from build123d import *

# Parameters (mm, degrees)
EXTRUDE1_DEPTH  = 5
SKETCH3_W       = 42
SKETCH3_H       = 47
EXTRUDE2_DEPTH  = 5
SKETCH4_W       = 34
SKETCH4_H       = 40
EXTRUDE3_DEPTH  = 3.2
EXTRUDE4_DEPTH  = 3
SKETCH6_R       = 1.5
EXTRUDE5_DEPTH  = 5
SKETCH7_R       = 1.5
EXTRUDE6_DEPTH  = 5
SKETCH8_W       = 6.381599337
SKETCH8_H       = 7
EXTRUDE7_DEPTH  = 5
SKETCH9_R       = 1.5
EXTRUDE8_DEPTH  = 5
FILLET1_R       = 5
FILLET2_R       = 2
SKETCH11_R      = 2
EXTRUDE10_DEPTH = 5
SKETCH15_R      = 13
EXTRUDE13_DEPTH = 4
SKETCH16_W      = 45
SKETCH16_H      = 40
EXTRUDE14_DEPTH = 3.5
SKETCH17_R      = 1.5
EXTRUDE16_DEPTH = 5
SKETCH18_R      = 1.5
EXTRUDE17_DEPTH = 5
SKETCH20_R      = 2
EXTRUDE19_DEPTH = 5
EXTRUDE24_START = -1.5
EXTRUDE24_DEPTH = 1.5
EXTRUDE25_START = -1.5
EXTRUDE25_DEPTH = 1.5
SKETCH27_R      = 1.5
EXTRUDE26_DEPTH = 5
SKETCH28_R      = 1.5
EXTRUDE27_DEPTH = 5
SKETCH29_R      = 4
EXTRUDE28_DEPTH = 3
SKETCH30_R      = 2
EXTRUDE29_DEPTH = 2
SKETCH14_R      = 1.25
EXTRUDE30_DEPTH = 5


with BuildPart() as part:
    # Sketch2 → Extrude1 (new body)
    with BuildSketch(Plane(origin=(0, 0, 0), x_dir=(1, 0, 0), z_dir=(0, 1, 0))):
        with BuildLine():
            Line((82.558104656, 20.227687844), (67.247468193, 10.284844268))
            Line((67.247468193, 10.284844268), (38.381599337, 54.73438437))
            Line((38.381599337, 54.73438437), (38.381599337, 66.73438437))
            Line((38.381599337, 66.73438437), (-38.381599337, 66.73438437))
            Line((-38.381599337, 66.73438437), (-38.381599337, 54.73438437))
            Line((-38.381599337, 54.73438437), (-67.247468193, 10.284844268))
            Line((-67.247468193, 10.284844268), (-82.558104656, 20.227687844))
            ThreePointArc((-82.558104656, 20.227687844), (-84.534361106, -8.884919378), (-76.54843921, -36.950459463))
            Line((-76.54843921, -36.950459463), (-63.639610307, -24.04163056))
            Line((-63.639610307, -24.04163056), (-24.04163056, -63.639610307))
            Line((-24.04163056, -63.639610307), (-36.950459463, -76.54843921))
            ThreePointArc((-36.950459463, -76.54843921), (0, -85), (36.950459463, -76.54843921))
            Line((36.950459463, -76.54843921), (24.04163056, -63.639610307))
            Line((24.04163056, -63.639610307), (63.639610307, -24.04163056))
            Line((63.639610307, -24.04163056), (76.54843921, -36.950459463))
            ThreePointArc((76.54843921, -36.950459463), (84.534361106, -8.884919378), (82.558104656, 20.227687844))
        make_face()
    extrude(amount=-EXTRUDE1_DEPTH)

    # Sketch3 → Extrude2 (cut)
    with BuildSketch(Plane(origin=(0, 0, 0), x_dir=(1, 0, 0), z_dir=(0, 1, 0))):
        with Locations((0, 48.23438437)):
            Rectangle(SKETCH3_W, SKETCH3_H)
    extrude(amount=-EXTRUDE2_DEPTH, mode=Mode.SUBTRACT)

    # Sketch4 → Extrude3 (cut)
    with BuildSketch(Plane(origin=(0, 0, 0), x_dir=(-1, 0, 0), z_dir=(0, 1, 0))):
        with Locations((0, -10.73438437)):
            Rectangle(SKETCH4_W, SKETCH4_H)
    extrude(amount=-EXTRUDE3_DEPTH, mode=Mode.SUBTRACT)

    # Sketch5 → Extrude4 (cut)
    with BuildSketch(Plane(origin=(0, 0, 0), x_dir=(1, 0, 0), z_dir=(0, 1, 0))):
        Polygon((43.470660758, -6.348358315), (62.76008382, 6.17833949), (43.697717595, 35.531809369), (24.408294532, 23.005111563), align=None)
    extrude4 = extrude(amount=-EXTRUDE4_DEPTH, mode=Mode.SUBTRACT)

    # Mirror1: Extrude4 across plane
    add(extrude4.mirror(Plane(origin=(0, 0, 0), x_dir=(0, 0, 1), z_dir=(1, 0, 0))), mode=Mode.SUBTRACT)

    # Sketch6 → Extrude5 (cut)
    with BuildSketch(Plane(origin=(0, 0, 0), x_dir=(1, 0, 0), z_dir=(0, 1, 0))):
        with Locations(Location((42.401256054, 43.036420449, 0), (0, 0, 270))):
            Circle(SKETCH6_R)
        with Locations(Location((60.918983244, 14.521621139, 0), (0, 0, 270))):
            Circle(SKETCH6_R)
        with Locations(Location((50.911688245, -32.526911935, 0), (0, 0, 270))):
            Circle(SKETCH6_R)
        with Locations(Location((32.526911935, -50.911688245, 0), (0, 0, 270))):
            Circle(SKETCH6_R)
    extrude5 = extrude(amount=-EXTRUDE5_DEPTH, mode=Mode.SUBTRACT)

    # Mirror2: Extrude5 across plane
    add(extrude5.mirror(Plane(origin=(0, 0, 0), x_dir=(0, 0, 1), z_dir=(1, 0, 0))), mode=Mode.SUBTRACT)

    # Sketch7 → Extrude6 (cut)
    with BuildSketch(Plane(origin=(0, 0, 0), x_dir=(-1, 0, 0), z_dir=(0, 1, 0))):
        with Locations(Location((-24, -63.73438437, 0), (0, 0, 90))):
            Circle(SKETCH7_R)
        with Locations(Location((-24, -27.73438437, 0), (0, 0, 90))):
            Circle(SKETCH7_R)
    extrude6 = extrude(amount=-EXTRUDE6_DEPTH, mode=Mode.SUBTRACT)

    # Mirror3: Extrude6 across plane
    add(extrude6.mirror(Plane(origin=(0, 0, 0), x_dir=(0, 0, 1), z_dir=(1, 0, 0))), mode=Mode.SUBTRACT)

    # Sketch8 → Extrude7 (cut)
    with BuildSketch(Plane(origin=(0, 0, 0), x_dir=(1, 0, 0), z_dir=(0, 1, 0))):
        with Locations((30.190799669, 65.23438437)):
            Rectangle(SKETCH8_W, SKETCH8_H)
    extrude7 = extrude(amount=-EXTRUDE7_DEPTH, mode=Mode.SUBTRACT)

    # Mirror4: Extrude7 across plane
    add(extrude7.mirror(Plane(origin=(0, 0, 0), x_dir=(0, 0, 1), z_dir=(1, 0, 0))), mode=Mode.SUBTRACT)

    # Sketch9 → Extrude8 (cut)
    with BuildSketch(Plane(origin=(0, 0, 0), x_dir=(1, 0, 0), z_dir=(0, 1, 0))):
        with Locations(Location((35.881599337, 60.13438437, 0), (0, 0, 270))):
            Circle(SKETCH9_R)
        with Locations(Location((35.881599337, 46.73438437, 0), (0, 0, 270))):
            Circle(SKETCH9_R)
    extrude8 = extrude(amount=-EXTRUDE8_DEPTH, mode=Mode.SUBTRACT)

    # Mirror5: Extrude8 across plane
    add(extrude8.mirror(Plane(origin=(0, 0, 0), x_dir=(0, 0, 1), z_dir=(1, 0, 0))), mode=Mode.SUBTRACT)

    # Fillet1
    fillet1_edges = [part.edges().sort_by_distance(p)[0] for p in [
        (76.54843921, -2.5, 36.950459463),
        (63.639610307, -2.5, 24.04163056),
        (24.04163056, -2.5, 63.639610307),
        (36.950459463, -2.5, 76.54843921),
        (-36.950459463, -2.5, 76.54843921),
        (-24.04163056, -2.5, 63.639610307),
        (-63.639610307, -2.5, 24.04163056),
        (-76.54843921, -2.5, 36.950459463),
        (-82.558104656, -2.5, -20.227687844),
        (-67.247468193, -2.5, -10.284844268),
        (-38.381599337, -2.5, -54.73438437),
        (38.381599337, -2.5, -54.73438437),
        (67.247468193, -2.5, -10.284844268),
        (82.558104656, -2.5, -20.227687844),
    ]]
    fillet(fillet1_edges, radius=FILLET1_R)

    # Fillet2
    fillet2_edges = [part.edges().sort_by_distance(p)[0] for p in [
        (-43.470660758, -1.5, 6.348358315),
        (-62.76008382, -1.5, -6.17833949),
        (-43.697717595, -1.5, -35.531809369),
        (-17, -1.6, 9.26561563),
        (17, -1.6, 9.26561563),
        (43.470660758, -1.5, 6.348358315),
        (24.408294532, -1.5, -23.005111563),
        (43.697717595, -1.5, -35.531809369),
        (62.76008382, -1.5, -6.17833949),
        (-24.408294532, -1.5, -23.005111563),
    ]]
    fillet(fillet2_edges, radius=FILLET2_R)

    # Sketch11 → Extrude10 (cut)
    with BuildSketch(Plane(origin=(0, 0, 0), x_dir=(1, 0, 0), z_dir=(0, 1, 0))):
        with Locations(Location((24.5, 36, 0), (0, 0, 270))):
            Circle(SKETCH11_R)
        with Locations(Location((-24.5, 36, 0), (0, 0, 270))):
            Circle(SKETCH11_R)
    extrude(amount=-EXTRUDE10_DEPTH, mode=Mode.SUBTRACT)

    # Sketch15 → Extrude13 (cut)
    with BuildSketch(Plane(origin=(0, 0, 0), x_dir=(1, 0, 0), z_dir=(0, 1, 0))):
        with Locations(Location((69, -13, 0), (0, 0, 270))):
            Circle(SKETCH15_R)
    extrude13 = extrude(amount=-EXTRUDE13_DEPTH, mode=Mode.SUBTRACT)

    # Mirror7: Extrude13 across plane
    add(extrude13.mirror(Plane(origin=(0, 0, 0), x_dir=(0, 0, 1), z_dir=(1, 0, 0))), mode=Mode.SUBTRACT)

    # Sketch16 → Extrude14 (cut)
    with BuildSketch(Plane(origin=(0, 0, 0), x_dir=(1, 0, 0), z_dir=(0, 1, 0))):
        with Locations((0, -75)):
            Rectangle(SKETCH16_W, SKETCH16_H)
    extrude(amount=-EXTRUDE14_DEPTH, mode=Mode.SUBTRACT)

    # Sketch17 → Extrude16 (cut)
    with BuildSketch(Plane(origin=(0, 0, 0), x_dir=(1, 0, 0), z_dir=(0, 1, 0))):
        with Locations(Location((25.5, -70, 0), (0, 0, 270))):
            Circle(SKETCH17_R)
        with Locations(Location((-25.5, -70, 0), (0, 0, 270))):
            Circle(SKETCH17_R)
    extrude(amount=-EXTRUDE16_DEPTH, mode=Mode.SUBTRACT)

    # Sketch18 → Extrude17 (cut)
    with BuildSketch(Plane(origin=(0, 0, 0), x_dir=(-1, 0, 0), z_dir=(0, 1, 0))):
        with Locations(Location((-11, 52, 0), (0, 0, 90))):
            Circle(SKETCH18_R)
        with Locations(Location((11, 52, 0), (0, 0, 90))):
            Circle(SKETCH18_R)
    extrude(amount=-EXTRUDE17_DEPTH, mode=Mode.SUBTRACT)

    # Sketch20 → Extrude19 (cut)
    with BuildSketch(Plane(origin=(0, 0, 0), x_dir=(1, 0, 0), z_dir=(0, 1, 0))):
        with Locations(Location((20.5, -2, 0), (0, 0, 270))):
            Circle(SKETCH20_R)
        with Locations(Location((-20.5, -2, 0), (0, 0, 270))):
            Circle(SKETCH20_R)
    extrude(amount=-EXTRUDE19_DEPTH, mode=Mode.SUBTRACT)

    # Sketch23 → Extrude24 (add)
    with BuildSketch(Plane.XZ.offset(5).offset(EXTRUDE24_START)):
        with BuildLine():
            Line((84.035839065, -12.766274034), (87.035839065, -12.766274034))
            ThreePointArc((87.035839065, -12.766274034), (87.519327499, 8.864668549), (82.708242384, 29.959333706))
            Line((82.708242384, 29.959333706), (79.545196737, 29.959333706))
            ThreePointArc((79.545196737, 29.959333706), (84.534361106, 8.884919378), (84.035839065, -12.766274034))
        make_face()
    extrude24 = extrude(amount=EXTRUDE24_DEPTH)

    # Mirror8: Extrude24 across plane
    add(extrude24.mirror(Plane(origin=(0, 0, 0), x_dir=(0, 0, 1), z_dir=(1, 0, 0))))

    # Sketch24 → Extrude25 (add)
    with BuildSketch(Plane.XZ.offset(5).offset(EXTRUDE25_START)):
        with BuildLine():
            Line((-29.959333706, 79.545196737), (-29.959333706, 82.545196737))
            ThreePointArc((-29.959333706, 82.545196737), (0, 87.8138439), (29.959333706, 82.545196737))
            Line((29.959333706, 82.545196737), (29.959333706, 79.545196737))
            ThreePointArc((29.959333706, 79.545196737), (0, 85), (-29.959333706, 79.545196737))
        make_face()
    extrude(amount=EXTRUDE25_DEPTH)

    # Sketch27 → Extrude26 (cut)
    with BuildSketch(Plane(origin=(0, 0, 0), x_dir=(1, 0, 0), z_dir=(0, 1, 0))):
        with Locations(Location((20, 21.73438437, 0), (0, 0, 270))):
            Circle(SKETCH27_R)
        with Locations(Location((-20, 21.73438437, 0), (0, 0, 270))):
            Circle(SKETCH27_R)
    extrude(amount=-EXTRUDE26_DEPTH, mode=Mode.SUBTRACT)

    # Sketch28 → Extrude27 (cut)
    with BuildSketch(Plane(origin=(0, 0, 0), x_dir=(1, 0, 0), z_dir=(0, 1, 0))):
        with Locations(Location((28.5, -8.6, 0), (0, 0, 270))):
            Circle(SKETCH28_R)
        with Locations(Location((-28.5, -8.6, 0), (0, 0, 270))):
            Circle(SKETCH28_R)
    extrude(amount=-EXTRUDE27_DEPTH, mode=Mode.SUBTRACT)

    # Sketch29 → Extrude28 (cut)
    with BuildSketch(Plane(origin=(0, 0, 0), x_dir=(1, 0, 0), z_dir=(0, 1, 0))):
        with Locations(Location((-79.5, 5, 0), (0, 0, 270))):
            Circle(SKETCH29_R)
        with Locations(Location((79.5, 5, 0), (0, 0, 270))):
            Circle(SKETCH29_R)
    extrude(amount=-EXTRUDE28_DEPTH, mode=Mode.SUBTRACT)

    # Sketch30 → Extrude29 (cut)
    with BuildSketch(Plane(origin=(0, -3, 0), x_dir=(1, 0, 0), z_dir=(0, 1, 0))):
        with Locations(Location((79.5, 5, 0), (0, 0, 270))):
            Circle(SKETCH30_R)
        with Locations(Location((-79.5, 5, 0), (0, 0, 270))):
            Circle(SKETCH30_R)
    extrude(amount=-EXTRUDE29_DEPTH, mode=Mode.SUBTRACT)

    # Sketch14 → Extrude30 (cut)
    with BuildSketch(Plane(origin=(0, 0, 0), x_dir=(1, 0, 0), z_dir=(0, 1, 0))):
        with Locations(Location((24.203535757, 14.52559661, 0), (0, 0, 270))):
            Circle(SKETCH14_R)
        with Locations(Location((29.649926107, 6.13889093, 0), (0, 0, 270))):
            Circle(SKETCH14_R)
        with Locations(Location((23.483016203, -16.411948391, 0), (0, 0, 270))):
            Circle(SKETCH14_R)
        with Locations(Location((16.411948391, -23.483016203, 0), (0, 0, 270))):
            Circle(SKETCH14_R)
        with Locations(Location((26.926730932, 10.33224377, 0), (0, 0, 270))):
            Circle(SKETCH14_R)
        with Locations(Location((32.373121282, 1.945538091, 0), (0, 0, 270))):
            Circle(SKETCH14_R)
    extrude30 = extrude(amount=-EXTRUDE30_DEPTH, mode=Mode.SUBTRACT)

    # Mirror9: Extrude30 across plane
    add(extrude30.mirror(Plane(origin=(0, 0, 0), x_dir=(0, 0, 1), z_dir=(1, 0, 0))), mode=Mode.SUBTRACT)


solid = part.part
CAD build for the part. Positions are in the model's coordinates, mm. A direction names the side the tool comes from. Give positions to 0.01 mm unless a question says otherwise; leave off trailing zeros. Answer in a Markdown table with one row per item. Add a question column.
Item 1: Mould opens along Z. For faces 1 (the face through (69.2, -2.5, 29.6)), 2 (the face through (73.94, -2.46, -14.63)), 3 (the face through (69, -4, 13)) say: +Z half, -Z half, draft (parallel to the pull), parting line (faces both ways), or undercut.
Item 2: Probe probe 1 along X at (y, z) = (-0.3, 22); probe 2 along X at (y, z) = (-2.3, 65.5); probe 3 along X at (y, z) = (-3.3, 27). List the from-to ranges inside material, lowest first.
Item 3: Tool access for faces 4 (the face through (27, -2, -64)), 5 (the face through (29.7, -2.5, 69.3)), 6 (the face through (84.5, -1.7, 9.2)), 7 (the face through (-53, -1.48, 0.16)): list every direction of +Z, -Z, +X, -X, +Y, -Y with a clear straight run to the whole face (end or side of a thin tool).
Item 4: Band-saw the part on A-A on z = 2. Give the number of separate pieces and of enclosed holes in the cut face, then the cut area to 3 significant figures.
Item 5: Drop flat-ended pins along their axis: P1, Ø2, axis at y = -1.5, z = 43, coming from the -X side; P2, Ø1.6, axis at x = 85.5, y = -4.5, coming from the -Z side; P3, Ø1.5, axis at y = -2, z = 5.5, coming from the +X side. Give the stop position or say it passes through.
Reply:
| question | item | result |
|---|---|---|
| 1 | face 1 | +Z half |
| 1 | face 2 | -Z half |
| 1 | face 3 | undercut |
| 2 | probe 1 | x = -82.1 to -78.38, -59.62 to 59.62, 78.38 to 82.1 |
| 2 | probe 2 | x = -26.47 to -22.5, 22.5 to 26.47 |
| 2 | probe 3 | x = -80.6 to -66.48, -60.8 to 60.8, 66.48 to 80.6 |
| 3 | face 4 | -Z, +Y, -Y |
| 3 | face 5 | +X, +Y, -Y |
| 3 | face 6 | +X, +Y |
| 3 | face 7 | +Y |
| 4 | separate pieces | 3 |
| 4 | enclosed holes | 0 |
| 4 | area | 542 mm^2 |
| 5 | P1 | stops at x = -45.68 |
| 5 | P2 | stops at z = -12.77 |
| 5 | P3 | stops at x = 84.87 |
